Model file for the job. Use its own axes, mm. Face numbers are marked on the shaded views. A direction names the side the tool comes from. Coordinates: 2 decimals unless noted, no trailing zeros. Write each loop counter-clockwise with the first axis right and the second up, starting at its lowest first coordinate (ties: lowest second). Pieces come first, ordered by that corner, then holes. Notation, with made-up numbers: M 44,11.5 L 64,11.5 A36 ccw 64,47.5 Z; hole C -25.5,-16.75 d5. An arc over 180 degrees is marked long. Put each result on its own line as item: value. Start each with the question number.
Q1. Cut at D-D (y = 12.75). Write the cut outline in (x, z), then the cut area to 3 significant figures.
Q2. Drop flat-ended pins along their axis: pin 1 (3 mm diameter, centred on x = 0, y = 13.5, fed in from -Z); pin 2 (1.4 mm diameter, centred on x = 1, z = -1, fed in from -Y); pin 3 (6 mm diameter, centred on x = -3, y = 0, fed in from +Z); pin 4 (1.2 mm diameter, centred on x = 0, z = 24.9, fed in from +Y). Give the stop position or say it passes through.
Q3. Cut at B-B (x = -4.75). Write the cut outline in (y, z).
Q4. Which spindle directions (+Z, -Z, +X, -X, +Y, -Y) get a long thin tool onto all of the face, cutting with end or side? Do the marked faces 1, 2, 3, 4 and 5. Say none if no direction does.
Q5. Drill centre lines: line 1 along Z through (x, y) = (0, 5.95); line 2 along X through (y, z) = (16.95, 5.9); line 3 along Y through (x, z) = (-4.25, 4.5). Where is each one in solid material? Low to high.
Q6. Cut at A-A (z = 24.9). Write the cut outline in (x, y).
Q7. Cut at C-C (y = 15.75). Write the cut outline in (x, z), then the cut area to 3 significant figures.
```python
from build123d import *

# Parameters (mm, degrees)
SKETCH1_W           = 11.8
SKETCH1_H           = 22.7
BOSS_EXTRUDE1_DEPTH = 22.5
BOSS_EXTRUDE2_DEPTH = 4
SKETCH3_R           = 2.3
SKETCH3_R_2         = 0.85
BOSS_EXTRUDE3_DEPTH = 3
SKETCH4_W           = 4.7
SKETCH4_H           = 2.5
BOSS_EXTRUDE4_DEPTH = 11.8
CUT_EXTRUDE1_REACH  = 35.365
SKETCH5_R           = 1


with BuildPart() as part:
    # Sketch1 → Boss-Extrude1 (new body)
    with BuildSketch(Plane.XY):
        Rectangle(SKETCH1_W, SKETCH1_H)
    extrude(amount=BOSS_EXTRUDE1_DEPTH)

    # Sketch2 → Boss-Extrude2 (add)
    with BuildSketch(Plane(origin=(0, 11.35, 0), x_dir=(1, 0, 0), z_dir=(0, 1, 0))):
        with BuildLine():
            Line((2.5, -12.2), (2.5, -11.244155686))
            ThreePointArc((2.5, -11.244155686), (0, 0), (-2.5, -11.244155686))
            Line((-2.5, -11.244155686), (-2.5, -12.2))
            ThreePointArc((-2.5, -12.2), (0, -14.7), (2.5, -12.2))
        make_face()
    extrude(amount=BOSS_EXTRUDE2_DEPTH)

    # Sketch3 → Boss-Extrude3 (add)
    with BuildSketch(Plane(origin=(0, 15.35, 0), x_dir=(1, 0, 0), z_dir=(0, 1, 0))):
        with Locations(Location((0, -5.9, 0), (0, 0, 270))):
            Circle(SKETCH3_R)
        with Locations(Location((0, -5.9, 0), (0, 0, 270))):
            Circle(SKETCH3_R_2, mode=Mode.SUBTRACT)
    extrude(amount=BOSS_EXTRUDE3_DEPTH)

    # Sketch4 → Boss-Extrude4 (add)
    with BuildSketch(Plane.ZY.offset(5.9)):
        with Locations((-2.35, 5.8)):
            Rectangle(SKETCH4_W, SKETCH4_H)
        with Locations((24.85, 5.8)):
            Rectangle(SKETCH4_W, SKETCH4_H)
    extrude(amount=-BOSS_EXTRUDE4_DEPTH)

    # Sketch5 → Cut-Extrude1 (cut, up to next)
    with BuildSketch(Plane(origin=(0, 7.05, 0), x_dir=(1, 0, 0), z_dir=(0, 1, 0)), mode=Mode.PRIVATE) as cut_extrude1_sk1:
        with Locations(Location((0, 2.4, 0), (0, 0, 180))):
            Circle(SKETCH5_R)
    cut_extrude1_tool1 = extrude(cut_extrude1_sk1.sketch, amount=-CUT_EXTRUDE1_REACH, mode=Mode.PRIVATE) & part.part
    # Sketch5 → Cut-Extrude1 (cut, up to next)
    with BuildSketch(Plane(origin=(0, 7.05, 0), x_dir=(1, 0, 0), z_dir=(0, 1, 0)), mode=Mode.PRIVATE) as cut_extrude1_sk2:
        with Locations(Location((0, -24.9, 0), (0, 0, 180))):
            Circle(SKETCH5_R)
    cut_extrude1_tool2 = extrude(cut_extrude1_sk2.sketch, amount=-CUT_EXTRUDE1_REACH, mode=Mode.PRIVATE) & part.part
    add(cut_extrude1_tool1.solids().sort_by_distance((0, 7.05, -2.4))[0], mode=Mode.SUBTRACT)
    add(cut_extrude1_tool2.solids().sort_by_distance((0, 7.05, 24.9))[0], mode=Mode.SUBTRACT)


solid = part.part
```
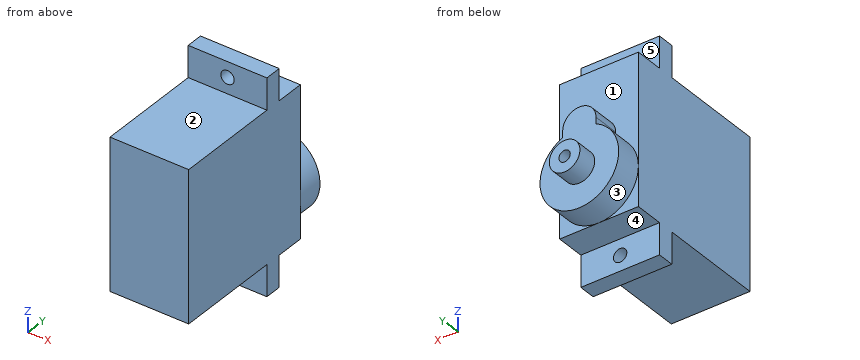
Computed values:
1. outline: M -2.5,11.24 A5.9 ccw long 2.5,11.24 L 2.5,12.2 A2.5 ccw -2.5,12.2 Z
1. area: 122 mm2
2. pin 1: z = 0
2. pin 2: y = 4.55
2. pin 3: z = 22.5
2. pin 4: through
3. outline: M -11.35,0 L 4.55,0 L 4.55,-4.7 L 7.05,-4.7 L 7.05,0 L 11.35,0 L 11.35,2.4 L 15.35,2.4 L 15.35,9.4 L 11.35,9.4 L 11.35,22.5 L 7.05,22.5 L 7.05,27.2 L 4.55,27.2 L 4.55,22.5 L -11.35,22.5 Z
4. face 1: +Z, +Y
4. face 2: +Z, +X, -X, -Y
4. face 3: +Y
4. face 4: -Z, +X, -X, +Y
4. face 5: +Z, +X, -X, +Y
5. line 1: -4.7 to -3.4, -1.4 to 23.9, 25.9 to 27.2
5. line 2: -2.3 to -0.85, 0.85 to 2.3
5. line 3: -11.35 to 15.35
6. outline: M -5.9,4.55 L -1,4.55 L -1,7.05 L -5.9,7.05 Z; M 1,4.55 L 5.9,4.55 L 5.9,7.05 L 1,7.05 Z
7. outline: C 0,5.9 d4.6; hole C 0,5.9 d1.7
7. area: 14.3 mm2
